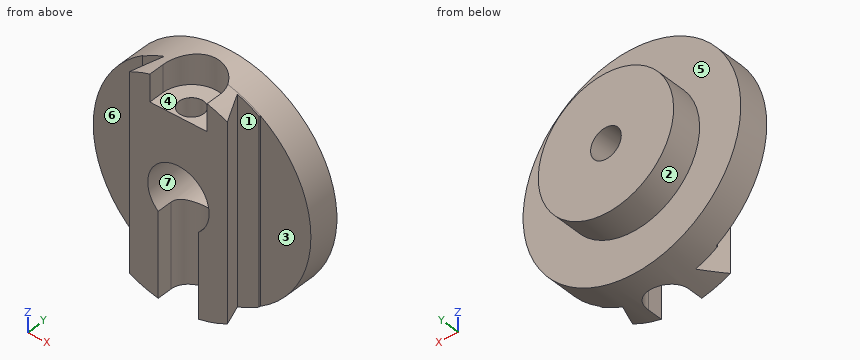
from build123d import *

# Parameters (mm, degrees)
Y_KSEKLIK_EKSTR_ZYON2_REACH                  = 120.76
Y_KSEKLIK_EKSTR_ZYON2_END_RADIUS             = 78
Y_KSEKLIK_EKSTR_ZYON2_DIRECTION_2_REACH      = 120.76
Y_KSEKLIK_EKSTR_ZYON2_DIRECTION_2_END_RADIUS = 78
KES_EKSTR_ZYON1_DEPTH                        = 22
M16_BO_LUKLU_DELIK2_D                        = 17.5
M16_BO_LUKLU_DELIK2_DEPTH                    = 55.999
M16_BO_LUKLU_DELIK2_CSINK_D                  = 17.55
M16_BO_LUKLU_DELIK2_CSINK_ANGLE              = 90
M16_BO_LUKLU_DELIK2_TIP                      = 5.257530416
KES_EKSTR_ZYON2_REACH                        = 187.785
KES_EKSTR_ZYON2_END_RADIUS                   = 22


with BuildPart() as part:
    # izim1 → D_nd_r1 (revolve)
    with BuildSketch(Plane.XY, mode=Mode.PRIVATE) as d_nd_r1_sk:
        Polygon((0, 0), (48.5, 0), (48.5, -22), (78, -22), (78, -44), (0, -44), align=None)
    revolve(d_nd_r1_sk.sketch.rotate(Axis((0, 0, 0), (0, -1, 0)), 90), axis=Axis((0, 0, 0), (0, -1, 0)))

    # Y_kseklik-Ekstr_zyon2: up to this cylinder (the profile starts inside it)
    y_kseklik_ekstr_zyon2_end = Plane(origin=(0, -54.257115, 0), z_dir=(0, 1, 0)) * Cylinder(Y_KSEKLIK_EKSTR_ZYON2_END_RADIUS, 398.52, mode=Mode.PRIVATE)
    # izim2 → Y_kseklik-Ekstr_zyon2 (add, up to the surface)
    with BuildSketch(Plane.XY, mode=Mode.PRIVATE) as y_kseklik_ekstr_zyon2_sk1:
        Polygon((-35, -64), (35, -64), (26.140154495, -45), (41.775578503, -45), (41.775578503, -44), (-41.775578503, -44), (-41.775578503, -45), (-26.140154495, -45), align=None)
    y_kseklik_ekstr_zyon2_tool1 = extrude(y_kseklik_ekstr_zyon2_sk1.sketch, amount=Y_KSEKLIK_EKSTR_ZYON2_REACH, mode=Mode.PRIVATE) & y_kseklik_ekstr_zyon2_end
    add(y_kseklik_ekstr_zyon2_tool1.solids().sort_by_distance((0, -54.257115, 0))[0])

    # Y_kseklik-Ekstr_zyon2 direction 2: up to this cylinder (the profile starts inside it)
    y_kseklik_ekstr_zyon2_direction_2_end = Plane(origin=(0, -54.257115, 0), z_dir=(0, 1, 0)) * Cylinder(Y_KSEKLIK_EKSTR_ZYON2_DIRECTION_2_END_RADIUS, 398.52, mode=Mode.PRIVATE)
    # izim2 → Y_kseklik-Ekstr_zyon2 direction 2 (add, up to the surface)
    with BuildSketch(Plane.XY, mode=Mode.PRIVATE) as y_kseklik_ekstr_zyon2_direction_2_sk1:
        Polygon((-35, -64), (35, -64), (26.140154495, -45), (41.775578503, -45), (41.775578503, -44), (-41.775578503, -44), (-41.775578503, -45), (-26.140154495, -45), align=None)
    y_kseklik_ekstr_zyon2_direction_2_tool1 = extrude(y_kseklik_ekstr_zyon2_direction_2_sk1.sketch, amount=-Y_KSEKLIK_EKSTR_ZYON2_DIRECTION_2_REACH, mode=Mode.PRIVATE) & y_kseklik_ekstr_zyon2_direction_2_end
    add(y_kseklik_ekstr_zyon2_direction_2_tool1.solids().sort_by_distance((0, -54.257115, 0))[0])

    # izim4 → Kes-D_nd_r1 (revolve, cut)
    with BuildSketch(Plane.XY, mode=Mode.PRIVATE) as kes_d_nd_r1_sk:
        Polygon((0, 0), (11, 0), (11, -21.868883424), (22, -22), (22, -64), (0, -64), align=None)
    revolve(kes_d_nd_r1_sk.sketch.rotate(Axis((0, 0, 0), (0, -1, 0)), 180), axis=Axis((0, 0, 0), (0, -1, 0)), mode=Mode.SUBTRACT)

    # izim6 → Kes-Ekstr_zyon1 (cut)
    with BuildSketch(Plane.XY.offset(78)):
        with BuildLine():
            Line((-20.5, -53), (-20.5, -64))
            Line((-20.5, -64), (0, -64))
            Line((0, -64), (20.5, -64))
            Line((20.5, -64), (20.5, -53))
            ThreePointArc((20.5, -53), (0, -32.5), (-20.5, -53))
        make_face()
    extrude(amount=-KES_EKSTR_ZYON1_DEPTH, mode=Mode.SUBTRACT)

    # M16 Bo_luklu Delik2
    with Locations(Plane(origin=(0, -53, 56), x_dir=(1, 0, 0), z_dir=(0, 0, 1))):
        with Locations((0, 0)):
            CounterSinkHole(M16_BO_LUKLU_DELIK2_D / 2, M16_BO_LUKLU_DELIK2_CSINK_D / 2, depth=M16_BO_LUKLU_DELIK2_DEPTH, counter_sink_angle=M16_BO_LUKLU_DELIK2_CSINK_ANGLE)
            with Locations((0, 0, -(M16_BO_LUKLU_DELIK2_DEPTH + M16_BO_LUKLU_DELIK2_TIP / 2))):  # 118° drill point
                Cone(0, M16_BO_LUKLU_DELIK2_D / 2, M16_BO_LUKLU_DELIK2_TIP, mode=Mode.SUBTRACT)

    # Kes-Ekstr_zyon2: up to this cylinder (the profile starts outside it)
    kes_ekstr_zyon2_end = Plane(origin=(0, -52.571949, 0), z_dir=(0, 1, 0)) * Cylinder(KES_EKSTR_ZYON2_END_RADIUS, 420.57, mode=Mode.PRIVATE)
    # izim10 → Kes-Ekstr_zyon2 (cut, up to the surface)
    with BuildSketch(Plane(origin=(0, 0, -78), x_dir=(-1, 0, 0), z_dir=(0, 0, -1)), mode=Mode.PRIVATE) as kes_ekstr_zyon2_sk1:
        with BuildLine():
            Line((-14.5, -53), (-14.5, -64))
            Line((-14.5, -64), (14.5, -64))
            Line((14.5, -64), (14.5, -53))
            ThreePointArc((14.5, -53), (0, -38.5), (-14.5, -53))
        make_face()
    kes_ekstr_zyon2_tool1 = extrude(kes_ekstr_zyon2_sk1.sketch, amount=-KES_EKSTR_ZYON2_REACH, mode=Mode.PRIVATE) - kes_ekstr_zyon2_end
    add(kes_ekstr_zyon2_tool1.solids().sort_by_distance((0, -52.571949, -78))[0], mode=Mode.SUBTRACT)


solid = part.part
Could you check a few things on this model? Use its own coordinates, in mm. Face numbers are marked on the shaded views. A direction names the side the tool comes from. Give positions to 0.01 mm unless a question says otherwise; leave off trailing zeros. Loops run counter-clockwise (first coordinate to the right, second up) from the corner with the lowest first, then second, coordinate; pieces in that order, holes last. Notation, with made-up numbers: (-22.5, 66) -> (29.5, 66) arc R25 ccw to (29.5, 103) -> close; hole circle Ø5 at (56.5, 60). An arc over 180 degrees is marked (long way). Answer as CSV lines item,"result". Start each with the question number.
(1) I need wall thicknesses on probe 1 along Z at (x, y) = (0, -34.5); probe 2 along Y at (x, z) = (0, 41.5); probe 3 along Y at (x, z) = (-45.5, 24). Which ranges of each line are inside material? Lowest first, please.
(2) If we section it at D-D on z = -39: Write out the boundary of the cut face in (x, y).
(3) I'm going to push flat-ended pins straight in: pin 1 Ø1 at (x, z) = (-44, 46.5) entering from +Y; pin 2 Ø5 at (x, z) = (-50.5, 18) entering from -Y; pin 3 Ø2 at (y, z) = (-36, -51.5) entering from -X; pin 4 Ø25 at (x, y) = (4, -42) entering from +Z. Where does each tip first touch, or does it pass through?
(4) We'd pull the mould along Y, two halves only. Please class the marked faces 1, 2 and 3: released by +Y, released by -Y, zero draft, split by the parting line, or undercut.
(5) If we section it at A-A on z = 0: Write out the boundary of the cut face in (x, y).
(6) If we section it at C-C on y = -29: Write out the boundary of the cut face in (x, z), then the cut area to 3 significant figures.
(7) If we section it at B-B on x = 0: Write out the boundary of the cut face in (y, z) (3 decimals).
(8) Which directions (+Z, -Z, +X, -X, +Y, -Y) give clear straight access to the entire face, cutting with the end or side of a thin tool? Please do the marked faces 4, 5, 6 and 7.
Computed:
1,probe 1,"z = -78 to -22, 22 to 56"
1,probe 2,"y = -64 to -61.75, -44.25 to 0"
1,probe 3,"y = -44 to -22"
2,outline,"(-67.55, -44) -> (-41.78, -44) -> (-41.78, -45) -> (-26.14, -45) -> (-35, -64) -> (-14.5, -64) -> (-14.5, -53) arc R14.5 cw to (14.5, -53) -> (14.5, -64) -> (35, -64) -> (26.14, -45) -> (41.78, -45) -> (41.78, -44) -> (67.55, -44) -> (67.55, -22) -> (28.83, -22) -> (28.83, 0) -> (-28.83, 0) -> (-28.83, -22) -> (-67.55, -22) -> close"
3,pin 1,"stops at y = -22"
3,pin 2,"stops at y = -44"
3,pin 3,"stops at x = -59.45"
3,pin 4,"stops at z = 78"
4,face 1,"undercut"
4,face 2,"zero draft"
4,face 3,"released by -Y"
5,outline,"(-78, -44) -> (-41.78, -44) -> (-41.78, -45) -> (-26.14, -45) -> (-35, -64) -> (-22, -64) -> (-22, -22) -> (-11, -21.87) -> (-11, 0) -> (-48.5, 0) -> (-48.5, -22) -> (-78, -22) -> close; (11, -21.87) -> (22, -22) -> (22, -64) -> (35, -64) -> (26.14, -45) -> (41.78, -45) -> (41.78, -44) -> (78, -44) -> (78, -22) -> (48.5, -22) -> (48.5, 0) -> (11, 0) -> close"
6,outline,"circle Ø156 at (0, 0); hole circle Ø44 at (0, 0)"
6,area,"17,600 mm2"
7,outline,"(-64, 22) -> (-61.75, 22) -> (-61.75, 55.975) -> (-61.775, 56) -> (-64, 56) -> close; (-44.25, 22) -> (-22, 22) -> (-21.869, 11) -> (0, 11) -> (0, 48.5) -> (-22, 48.5) -> (-22, 78) -> (-32.5, 78) -> (-32.5, 56) -> (-44.225, 56) -> (-44.25, 55.975) -> close; (-38.5, -78) -> (-22, -78) -> (-22, -48.5) -> (0, -48.5) -> (0, -11) -> (-21.869, -11) -> (-22, -22) -> (-38.5, -22) -> close"
8,face 4,"+Z, -Y"
8,face 5,"+Y"
8,face 6,"+Z, -Z, -X, -Y"
8,face 7,"-Y"
